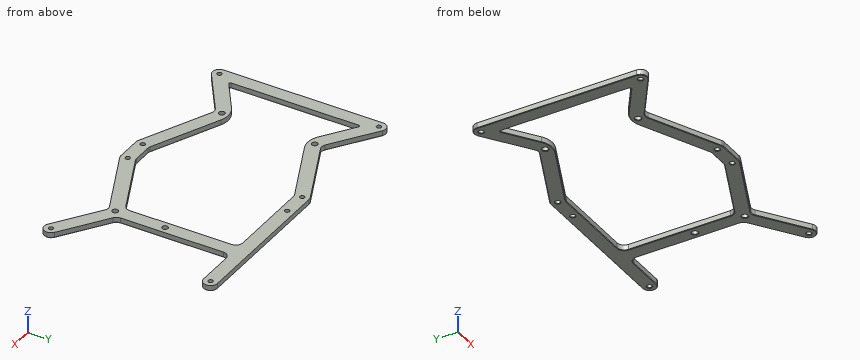
```python
from build123d import *

# Parameters (mm, degrees)
F3_DEPTH = 4
F0_R     = 2.1
F1_R     = 1.7
F4_DEPTH = 4.001
F5_SIZE  = 0.4


with BuildPart() as f3:
    # F2 (on Top) → F3 (new body)
    with BuildSketch(Plane.XY):
        with BuildLine():
            ThreePointArc((-106, -57.5), (-103.322028, -61.928113), (-98.156725, -61.612881))
            Line((-98.156725, -61.612881), (-66.331389, -39.611712))
            ThreePointArc((-66.331389, -39.611712), (-63.933431, -38.744463), (-61.419649, -39.172511))
            Line((-61.419649, -39.172511), (-11.068465, -62.052082))
            ThreePointArc((-11.068465, -62.052082), (-10.058204, -62.386738), (-9, -62.5))
            Line((-9, -62.5), (9, -62.5))
            ThreePointArc((9, -62.5), (10.058204, -62.386738), (11.068465, -62.052082))
            Line((11.068465, -62.052082), (61.419649, -39.172511))
            ThreePointArc((61.419649, -39.172511), (63.933431, -38.744463), (66.331389, -39.611712))
            Line((66.331389, -39.611712), (98.156725, -61.612881))
            ThreePointArc((98.156725, -61.612881), (105.112881, -60.343275), (103.843275, -53.387119))
            Line((103.843275, -53.387119), (71.156725, -30.790585))
            ThreePointArc((71.156725, -30.790585), (69.571887, -28.999732), (69, -26.677705))
            Line((69, -26.677705), (69, 47.5))
            ThreePointArc((69, 47.5), (70.464466, 51.035534), (74, 52.5))
            Line((74, 52.5), (101, 52.5))
            ThreePointArc((101, 52.5), (106, 57.5), (101, 62.5))
            Line((101, 62.5), (-9, 62.5))
            ThreePointArc((-9, 62.5), (-10.058204, 62.386738), (-11.068465, 62.052082))
            Line((-11.068465, 62.052082), (-61.419649, 39.172511))
            ThreePointArc((-61.419649, 39.172511), (-63.933431, 38.744463), (-66.331389, 39.611712))
            Line((-66.331389, 39.611712), (-98.156725, 61.612881))
            ThreePointArc((-98.156725, 61.612881), (-103.322028, 61.928113), (-106, 57.5))
            Line((-106, 57.5), (-106, -57.5))
        make_face()
        with BuildLine():
            Line((-8.903005, -52.052082), (-57.282718, -30.068347))
            ThreePointArc((-57.282718, -30.068347), (-64.824064, -28.784204), (-72.017939, -31.385951))
            Line((-72.017939, -31.385951), (-94.431345, -46.880559))
            ThreePointArc((-94.431345, -46.880559), (-95.464406, -46.943606), (-96, -46.057983))
            Line((-96, -46.057983), (-96, 46.057983))
            ThreePointArc((-96, 46.057983), (-95.464406, 46.943606), (-94.431345, 46.880559))
            Line((-94.431345, 46.880559), (-72.017939, 31.385951))
            ThreePointArc((-72.017939, 31.385951), (-64.824064, 28.784204), (-57.282718, 30.068347))
            Line((-57.282718, 30.068347), (-8.903005, 52.052082))
            ThreePointArc((-8.903005, 52.052082), (-7.892743, 52.386738), (-6.83454, 52.5))
            Line((-6.83454, 52.5), (54, 52.5))
            ThreePointArc((54, 52.5), (57.535534, 51.035534), (59, 47.5))
            Line((59, 47.5), (59, -26.068021))
            ThreePointArc((59, -26.068021), (58.203708, -28.775204), (56.068465, -30.620103))
            Line((56.068465, -30.620103), (8.903005, -52.052082))
            ThreePointArc((8.903005, -52.052082), (7.892743, -52.386738), (6.83454, -52.5))
            Line((6.83454, -52.5), (-6.83454, -52.5))
            ThreePointArc((-6.83454, -52.5), (-7.892743, -52.386738), (-8.903005, -52.052082))
        make_face(mode=Mode.SUBTRACT)
    extrude(amount=F3_DEPTH)

    # F0 (on Top) + F1 (on Top) → F4 (cut, through all)
    with BuildSketch(Plane.XY):
        with Locations((-64, 33.5)):
            Circle(F0_R)
        with Locations((-64, -33.5)):
            Circle(F0_R)
        with Locations((64, -33.5)):
            Circle(F0_R)
        with Locations((64, 2.5)):
            Circle(F0_R)
    with BuildSketch(Plane.XY):
        with Locations((-101, -57.5)):
            Circle(F1_R)
        with Locations((-101, 57.5)):
            Circle(F1_R)
        with Locations((-9, 57.5)):
            Circle(F1_R)
        with Locations((9, 57.5)):
            Circle(F1_R)
        with Locations((-9, -57.5)):
            Circle(F1_R)
        with Locations((9, -57.5)):
            Circle(F1_R)
        with Locations((101, -57.5)):
            Circle(F1_R)
        with Locations((101, 57.5)):
            Circle(F1_R)
    extrude(amount=F4_DEPTH, mode=Mode.SUBTRACT)

    # F5
    f5_edges = [f3.edges().sort_by_distance(p)[0] for p in [
        (-36.244057, 50.612297, 0),
        (-10.058204, 62.386738, 0),
        (-63.933431, 38.744463, 0),
        (46, 62.5, 0),
        (-82.244057, 50.612297, 0),
        (106, 57.5, 0),
        (-103.322028, 61.928113, 0),
        (87.5, 52.5, 0),
        (-106, 0, 0),
        (70.464466, 51.035534, 0),
        (-103.322028, -61.928113, 0),
        (69, 10.411148, 0),
        (-82.244057, -50.612297, 0),
        (69.571887, -28.999732, 0),
        (-63.933431, -38.744463, 0),
        (87.5, -42.088852, 0),
        (-36.244057, -50.612297, 0),
        (105.112881, -60.343275, 0),
        (-10.058204, -62.386738, 0),
        (82.244057, -50.612297, 0),
        (0, -62.5, 0),
        (63.933431, -38.744463, 0),
        (10.058204, -62.386738, 0),
        (36.244057, -50.612297, 0),
        (-102.7, -57.5, 0),
        (-66.1, -33.5, 0),
        (-10.7, -57.5, 0),
        (-33.092862, -41.060215, 0),
        (-7.892743, -52.386738, 0),
        (-64.824064, -28.784204, 0),
        (0, -52.5, 0),
        (-83.224642, -39.133255, 0),
        (7.892743, -52.386738, 0),
        (-95.464406, -46.943606, 0),
        (32.485735, -41.336093, 0),
        (-96, 0, 0),
        (58.203708, -28.775204, 0),
        (-95.464406, 46.943606, 0),
        (59, 10.715989, 0),
        (-83.224642, 39.133255, 0),
        (57.535534, 51.035534, 0),
        (-64.824064, 28.784204, 0),
        (23.58273, 52.5, 0),
        (-33.092862, 41.060215, 0),
        (-7.892743, 52.386738, 0),
        (7.3, -57.5, 0),
        (99.3, -57.5, 0),
        (61.9, -33.5, 0),
        (-66.1, 33.5, 0),
        (-102.7, 57.5, 0),
        (-10.7, 57.5, 0),
        (61.9, 2.5, 0),
        (7.3, 57.5, 0),
        (99.3, 57.5, 0),
    ]]
    chamfer(f5_edges, length=F5_SIZE)


solid = f3.part
```
Read the model definition and answer for the solid it produces. Units are mm, in the model's axes. Coordinates: 2 decimals unless noted, no trailing zeros. Loops run counter-clockwise (first coordinate to the right, second up) from the corner with the lowest first, then second, coordinate; pieces in that order, holes last. Notation, with made-up numbers: (76.25, -4.5) - (83.25, -4.5) arc R35 ccw to (83.25, 29.5) - close; hole circle Ø1 at (77.5, -6.75). An arc over 180 degrees is marked (long way). Answer in a Markdown table with one row per item.
1. Find section B-B, the plane y = 2.5. Write down the section's boundary in (x, z), then the cut area to 3 significant figures.
Conclusion:
| item | result |
|---|---|
| outline | (-106, 0.4) - (-105.6, 0) - (-96.4, 0) - (-96, 0.4) - (-96, 4) - (-106, 4) - close; (59, 0.4) - (59.4, 0) - (61.5, 0) - (61.9, 0.4) - (61.9, 4) - (59, 4) - close; (66.1, 0.4) - (66.5, 0) - (68.6, 0) - (69, 0.4) - (69, 4) - (66.1, 4) - close |
| area | 62.7 mm² |
2. Given pin 1 (1.8 mm diameter, centred on y = 3, z = 1.5, fed in from +X); pin 2 (1.8 mm diameter, centred on x = 86.5, z = 2.5, fed in from -Y), each flat-ended and moving along its own axis, determine where each tip first touches the part or whether it passes through.
Conclusion:
| item | result |
|---|---|
| pin 1 | stops at x = 69 |
| pin 2 | stops at y = -54.18 |
3. Find section D-D, the plane z = 2.7. Count the separate pieces of the cut face and the enclosed holes in it, then the cut area to 3 significant figures.
Conclusion:
| item | result |
|---|---|
| separate pieces | 1 |
| enclosed holes | 13 |
| area | 6,300 mm² |
4. Find section C-C, the plane x = 92. Write down the section's boundary in (y, z).
Conclusion:
| item | result |
|---|---|
| outline | (-57.36, 0.4) - (-56.87, 0) - (-45.69, 0) - (-45.2, 0.4) - (-45.2, 4) - (-57.36, 4) - close; (52.5, 0.4) - (52.9, 0) - (62.1, 0) - (62.5, 0.4) - (62.5, 4) - (52.5, 4) - close |
5. Straight lines are drawn through the part: line 1 (Y direction, x = 64, z = 1.95); line 2 (Y direction, x = -9, z = 2.8); line 3 (Y direction, x = -64, z = 1.45). For each, find the intervals that lie inside material, in ascending order.
Conclusion:
| item | result |
|---|---|
| line 1 | y = -38.75 to -35.6, -31.4 to 0.4, 4.6 to 62.5 |
| line 2 | y = -62.5 to -59.2, -55.8 to -52.01, 52.01 to 55.8, 59.2 to 62.5 |
| line 3 | y = -38.75 to -35.6, -31.4 to -28.73, 28.73 to 31.4, 35.6 to 38.75 |
6. Find section A-A, the plane y = -11. Write down the section's boundary in (x, z), then the cut area to 3 significant figures.
Conclusion:
| item | result |
|---|---|
| outline | (-106, 0.4) - (-105.6, 0) - (-96.4, 0) - (-96, 0.4) - (-96, 4) - (-106, 4) - close; (59, 0.4) - (59.4, 0) - (68.6, 0) - (69, 0.4) - (69, 4) - (59, 4) - close |
| area | 79.7 mm² |
